Geometry check sheet. Reference: drawing and pictorial views, mm from the part's lowest x, y, z. A direction names the side the tool comes from. Round coordinates to 2 decimals unless told otherwise and drop trailing zeros. Write each loop counter-clockwise with the first axis right and the second up, starting at its lowest first coordinate (ties: lowest second). Pieces come first, ordered by that corner, then holes. Notation, with made-up numbers: (-8, -28.5) -> (-4, -28.5) arc R14 cw to (-4, -19.5) -> close; hole circle Ø8 at (59.5, 2.25). An arc over 180 degrees is marked (long way). Answer as a JSON object with one key per item and string values. Group by question number.
(1) Sectioned sample at A-A on z = 18. Record the cut outline in (x, y).
(2) Sectioned sample at B-B on x = 50.5. Record the cut outline in (y, z).
(3) Scan lines: L1, parallel to X at y = 11.5, z = 11; L2, parallel to Y at x = 38, z = 1.5. Record each from-to range of solid material in increasing order. Write a range as from..to.
(4) Sectioned sample at C-C on x = 14.5. Record the cut outline in (y, z) (1 decimal), and give its area (3 significant figures).
(5) Gauge pin test, flat ends, axial feed: pin 1 Ø10 at (y, z) = (26, 15) entering from +X; pin 2 Ø1 at (y, z) = (9.5, 18) entering from +X; pin 3 Ø1.4 at (x, y) = (51, 30) entering from +Z; pin 4 Ø3.5 at (x, z) = (51, 12) entering from -Y. Record the tip position at first contact, or that the pin passes through.
(6) Set-up check for the marked faces 1, 2, 3, 4 and 5: record each of +Z, -Z, +X, -X, +Y, -Y from which the full face is reachable in a straight line by a thin tool's end or side.
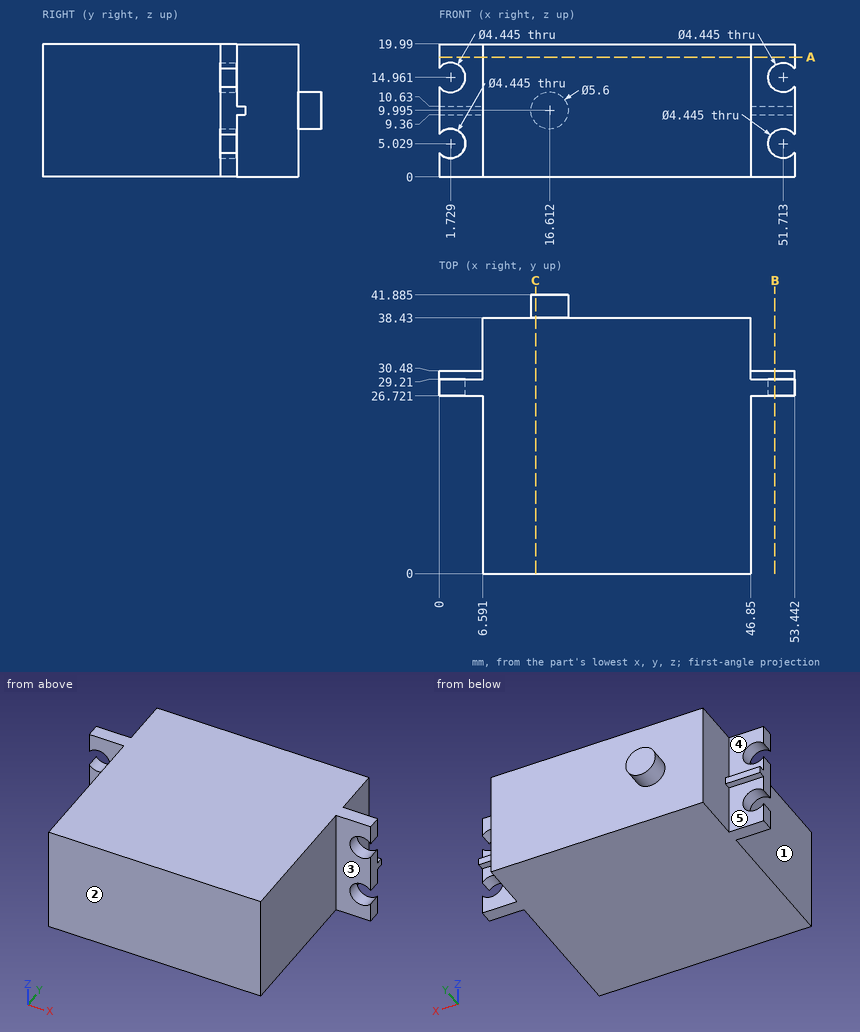
Computed values:
{
 "1": {"outline": "(0, 26.72) -> (6.59, 26.72) -> (6.59, 0) -> (46.85, 0) -> (46.85, 26.72) -> (53.44, 26.72) -> (53.44, 29.21) -> (46.85, 29.21) -> (46.85, 38.43) -> (6.59, 38.43) -> (6.59, 29.21) -> (0, 29.21) -> close"},
 "2": {"outline": "(26.72, 0) -> (29.21, 0) -> (29.21, 3.17) -> (26.72, 3.17) -> close; (26.72, 6.89) -> (29.21, 6.89) -> (29.21, 9.36) -> (30.48, 9.36) -> (30.48, 10.63) -> (29.21, 10.63) -> (29.21, 13.1) -> (26.72, 13.1) -> close; (26.72, 16.82) -> (29.21, 16.82) -> (29.21, 19.99) -> (26.72, 19.99) -> close"},
 "3": {"L1": "6.59..46.85", "L2": "0..38.43"},
 "4": {"outline": "(0, 0) -> (38.4, 0) -> (38.4, 8.2) -> (41.9, 8.2) -> (41.9, 11.8) -> (38.4, 11.8) -> (38.4, 20) -> (0, 20) -> close", "area": "781 mm2"},
 "5": {"pin 1": "x = 53.44", "pin 2": "x = 46.85", "pin 3": "z = 10.63", "pin 4": "y = 26.72"},
 "6": {"face 1": "+Z, -Z, -X, -Y", "face 2": "+Z, -Z, +X, -X, -Y", "face 3": "+Z, -Z, +X, -Y", "face 4": "+Z, -X, +Y", "face 5": "-Z, -X, +Y"}
}
